Source: CAD feature listing. Evaluate the final solid. Frame: model axes, mm. Face numbers are marked on the shaded views. A direction names the side the tool comes from. Round coordinates to 2 decimals unless told otherwise and drop trailing zeros. Order: outer loops, then holes, each group sorted by start corner. A loop starts at its lowest first (then second) coordinate and runs counter-clockwise, first axis right, second up. Notation, with made-up numbers: (-8, -38.75) - (36, -38.75) arc R16 ccw to (36, -21.75) - close; hole circle Ø9 at (26.25, 42.25). An arc over 180 degrees is marked (long way). Put each result on its own line as item: value. Start each with the question number.
1) Section B-B on y = 48.5. Output: boundary loops of the cut face in (x, z).
2) Access query for the marked faces 5 and 6. Directions: +Z, -Z, +X, -X, +Y, -Y. A direction counts if a zero-diameter tool reaches every point of the face in a straight line with its end or side. Return the directions, or none.
3) Line query: probe 1 along X at (y, z) = (0, 35.5); probe 2 along Z at (x, y) = (-24.5, -10); probe 3 along Z at (x, y) = (-7.5, 3.5). Output: solid intervals per line, ascending. Write a range as [from, to].
4) Section C-C on x = 27. Output: boundary loops of the cut face in (y, z).
5) Mould query, pull axis X, two halves, no side actions, for the marked faces 1, 2, 3 and 4. Classes: +X half, -X half, draft (parallel to the pull), parting line (faces both ways), or undercut.
6) Section D-D on z = 51.5. Output: boundary loops of the cut face in (x, y), then the cut area to 3 significant figures.
7) Section A-A on z = 12. Output: boundary loops of the cut face in (x, y).
8) Contact query for flat-ended pins moving along their axis: P1, Ø21, axis at y = 10.5, z = 7.5, coming from the +X side; P2, Ø5, axis at y = 59.5, z = 36.5, coming from the +X side; P3, Ø19, axis at x = -1.5, y = 11.5, coming from the +Z side. Output: stop coordinate, or through.
```python
from build123d import *

# Parameters (mm, degrees)
F0_R     = 63.5
F0_R_2   = 31.75
F0_R_3   = 19.05
F1_DEPTH = 19.05
F2_DEPTH = 57.15
F3_DEPTH = 31.75
F4_DEPTH = 25.4


with BuildPart() as f1:
    # F0 (on Top) → F1 (new body)
    with BuildSketch(Plane.XY):
        with BuildLine():
            ThreePointArc((0, 76.2), (53.881537, 53.881537), (76.2, 0))
            ThreePointArc((76.2, 0), (53.881537, -53.881537), (0, -76.2))
            Line((0, -76.2), (107.95, -76.2))
            ThreePointArc((107.95, -76.2), (127, -57.15), (107.95, -38.1))
            Line((107.95, -38.1), (107.95, 38.1))
            ThreePointArc((107.95, 38.1), (127, 57.15), (107.95, 76.2))
            Line((107.95, 76.2), (0, 76.2))
        make_face()
        with BuildLine():
            ThreePointArc((0, -76.2), (-76.2, 0), (0, 76.2))
            Line((0, 76.2), (-107.95, 76.2))
            ThreePointArc((-107.95, 76.2), (-126.996003, 57.540236), (-108.730309, 38.115988))
            Line((-108.730309, 38.115988), (-107.95, -38.1))
            ThreePointArc((-107.95, -38.1), (-127, -57.15), (-107.95, -76.2))
            Line((-107.95, -76.2), (0, -76.2))
        make_face()
        with BuildLine():
            ThreePointArc((0, -76.2), (53.881537, -53.881537), (76.2, 0))
            ThreePointArc((76.2, 0), (53.881537, 53.881537), (0, 76.2))
            ThreePointArc((0, 76.2), (-76.2, 0), (0, -76.2))
        make_face()
        Circle(F0_R, mode=Mode.SUBTRACT)
        Circle(F0_R)
        Circle(F0_R_2, mode=Mode.SUBTRACT)
        Circle(F0_R_2)
        Circle(F0_R_3, mode=Mode.SUBTRACT)
        Circle(F0_R_3)
    extrude(amount=F1_DEPTH)

    # F0 (on Top) → F2 (join)
    with BuildSketch(Plane.XY):
        with BuildLine():
            ThreePointArc((0, -76.2), (53.881537, -53.881537), (76.2, 0))
            ThreePointArc((76.2, 0), (53.881537, 53.881537), (0, 76.2))
            ThreePointArc((0, 76.2), (-76.2, 0), (0, -76.2))
        make_face()
        Circle(F0_R, mode=Mode.SUBTRACT)
    extrude(amount=F2_DEPTH)

    # F0 (on Top) → F3 (join)
    with BuildSketch(Plane.XY):
        Circle(F0_R_2)
        Circle(F0_R_3, mode=Mode.SUBTRACT)
    extrude(amount=F3_DEPTH)

    # F0 (on Top) → F4 (join)
    with BuildSketch(Plane.XY):
        Circle(F0_R_3)
    extrude(amount=F4_DEPTH)


solid = f1.part
```
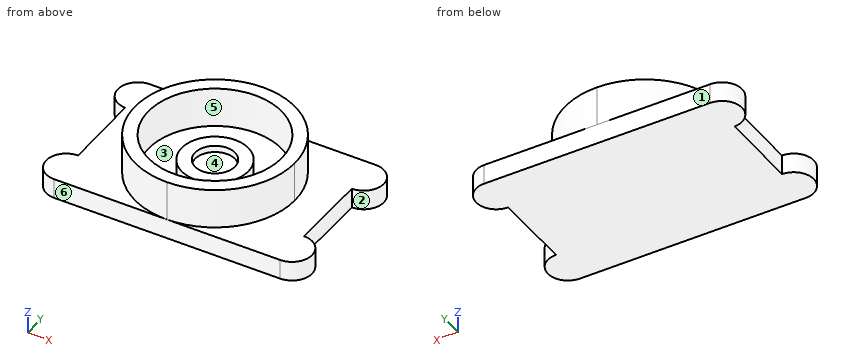
Answer sheet:
1. outline: (-124.92, 0) - (124.92, 0) - (124.92, 19.05) - (58.77, 19.05) - (58.77, 57.15) - (40.99, 57.15) - (40.99, 19.05) - (-40.99, 19.05) - (-40.99, 57.15) - (-58.77, 57.15) - (-58.77, 19.05) - (-124.92, 19.05) - close
2. face 5: +Z
2. face 6: +Z, -Z, +X, -X, -Y
3. probe 1: [-76.2, -63.5], [63.5, 76.2]
3. probe 2: [0, 31.75]
3. probe 3: [0, 25.4]
4. outline: (-76.2, 0) - (76.2, 0) - (76.2, 19.05) - (71.26, 19.05) - (71.26, 57.15) - (57.47, 57.15) - (57.47, 19.05) - (16.71, 19.05) - (16.71, 31.75) - (-16.71, 31.75) - (-16.71, 19.05) - (-57.47, 19.05) - (-57.47, 57.15) - (-71.26, 57.15) - (-71.26, 19.05) - (-76.2, 19.05) - close
5. face 1: draft
5. face 2: +X half
5. face 3: undercut
5. face 4: undercut
6. outline: (0, -76.2) arc R76.2 ccw to (76.2, 0) arc R76.2 ccw (long way) to start; hole circle Ø127 at (0, 0)
6. area: 5,570 mm^2
7. outline: (-108.73, 38.12) - (-107.95, -38.1) arc R19.05 ccw to (-107.95, -76.2) - (107.95, -76.2) arc R19.05 ccw to (107.95, -38.1) - (107.95, 38.1) arc R19.05 ccw to (107.95, 76.2) - (-107.95, 76.2) arc R19.05 ccw to start
8. P1: x = 107.95
8. P2: x = 50.57
8. P3: z = 31.75
